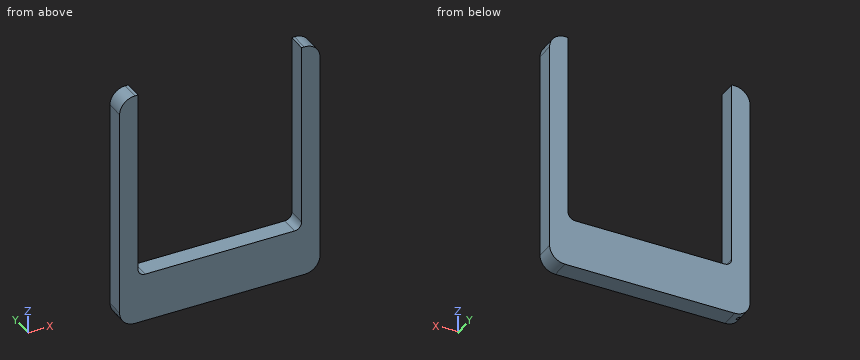
Autodesk Fusion 360 part; units mm, degrees
sketch "Sketch1" plane through (0, 0, 0) normal (0, 1, 0) x (1, 0, 0)
  line L0 (-207.5, 295) -> (207.5, 295)
  line L1 (245, 257.5) -> (245, -257.5)
  line L2 (-245, -257.5) -> (-245, 257.5)
  arc A0 (-207.5, 295) -> (-245, 257.5) centre (-207.5, 257.5) ccw
  arc A1 (245, 257.5) -> (207.5, 295) centre (207.5, 257.5) ccw
  arc A2 (207.5, -295) -> (245, -257.5) centre (207.5, -257.5) ccw
  arc A3 (-245, -257.5) -> (-207.5, -295) centre (-207.5, -257.5) ccw
  line L3 (-207.5, -295) -> (207.5, -295)
  line L4 (-207.5, 257.5) -> (207.5, -257.5) construction
  line L5 (-207.5, -257.5) -> (207.5, 257.5) construction
  point P0 (-245, 295)
  point P1 (245, 295)
  point P2 (-245, -523.5619)
  dimension "d2" = 490
  dimension "d6" = 37.5
  dimension "d10" = 590
extrude "Extrude1" add sketch "Sketch1" along normal blind 4
equation "d2 = 400 mm + 45 mm + 45 mm"
equation "d10 = 500.00 mm + 45 mm + 45 mm"

Autodesk Fusion 360 part; units mm, degrees
sketch "Sketch1" plane through (0, 0, 0) normal (0, 1, 0) x (1, 0, 0)
  line L0 (0, 0) -> (35, 0)
  line L1 (35, 0) -> (0, -35)
  line L2 (0, -35) -> (0, 0)
  dimension "d1" = 35
  dimension "d2" = 35
extrude "Extrude1" add sketch "Sketch1" along normal blind 45
sketch "Sketch2" plane through (0, 0, 0) normal (-1, 0, 0) x (0, 0, 1)
  line L0 (0, 0) -> (35, 0)
  line L1 (35, 0) -> (35, 45)
  line L2 (35, 45) -> (0, 45)
  line L3 (0, 45) -> (0, 0)
  line L4 (0, 45) -> (35, 0) construction
  circle A0 centre (17.5, 22.5) radius 4.5
  dimension "d5" = 9
extrude "Extrude2" cut sketch "Sketch2" against normal blind 110 contours A0
sketch "Sketch3" plane through (0, 0, 0) normal (0, 0, -1) x (-1, 0, 0)
  line L0 (-35, 0) -> (0, 0)
  line L1 (0, 0) -> (0, 45)
  line L2 (0, 45) -> (-35, 45)
  line L3 (-35, 45) -> (-35, 0)
  line L4 (0, 45) -> (-35, 0) construction
  circle A0 centre (-17.5, 22.5) radius 4.5
  point P0 (0, 22.5)
  dimension "d8" = 9
extrude "Extrude3" cut sketch "Sketch3" against normal blind 45 contours A0
sketch "Sketch4" plane through (0, 0, 0) normal (0, 0, -1) x (-1, 0, 0)
  circle A0 centre (-17.5, 22.5) radius 4.5
  line L0 (-35, 0) -> (0, 0)
  line L1 (0, 0) -> (0, 45)
  line L2 (0, 45) -> (-35, 45)
  line L3 (-35, 45) -> (-35, 0)
  point P0 (0, 22.5)

Autodesk Fusion 360 part; units mm, degrees
sketch "Sketch1" plane through (0, 0, 0) normal (0, 1, 0) x (1, 0, 0)
  line L0 (37.5, 0) -> (452.5, 0)
  line L1 (490, -37.5) -> (490, -552.7439)
  line L2 (0, -552.5) -> (0, -37.5)
  line L3 (445, -590) -> (445, -137.5)
  line L4 (427.5, -120) -> (62.5, -120)
  line L5 (45, -137.5) -> (45, -590)
  arc A0 (37.5, 0) -> (0, -37.5) centre (37.5, -37.5) ccw
  arc A1 (490, -37.5) -> (452.5, 0) centre (452.5, -37.5) ccw
  arc A2 (451.1619, -590.22) -> (490, -552.7439) centre (452.5, -552.7439) ccw
  arc A3 (0, -552.5) -> (37.5, -590) centre (37.5, -552.5) ccw
  arc A4 (62.5, -120) -> (45, -137.5) centre (62.5, -137.5) ccw
  arc A5 (445, -137.5) -> (427.5, -120) centre (427.5, -137.5) ccw
  line L6 (445, -590) -> (451.1619, -590.22)
  line L7 (37.5, -590) -> (45, -590)
  point P0 (490, 0)
  dimension "d1" = 45
  dimension "width" = 490
  dimension "d4" = 45
  dimension "d5" = 120
  dimension "d6" = 37.5
  dimension "d9" = 17.5
  dimension "length" = 590
  dimension "d11" = 590
extrude "Extrude1" add sketch "Sketch1" along normal blind 4
ref_plane "WorkPlane1" through (245, 0, 0) normal (1, 0, 0) x (0, 1, 0)
equation "width = 400 mm + 45 mm + 45 mm"
equation "length = 500.00 mm + 45 mm + 45 mm"
equation "d11 = length"
equation "d12 = width / 2"
Verification items for the finished model (mm, model axes). Coordinates: 2 decimals unless noted, no trailing zeros. Loops run counter-clockwise (first coordinate to the right, second up) from the corner with the lowest first, then second, coordinate; pieces in that order, holes last. Notation, with made-up numbers: (15.25, 73) -> (26.25, 73) arc R15 ccw to (26.25, 85) -> close; hole circle Ø5 at (64, 42). An arc over 180 degrees is marked (long way). Answer as CSV lines item,"result".
1) Cross-section at B-B, the plane x = 359. Record the cut outline in (y, z), then the cut area to 3 significant figures.
Found:
outline,"(0, 0) -> (45, 0) -> (45, 120) -> (0, 120) -> close"
area,"5,400 mm2"
2) Cross-section at A-A, the plane z = 364. Record the cut outline in (x, y), then the cut area to 3 significant figures.
Found:
outline,"(0, 0) -> (45, 0) -> (45, 45) -> (0, 45) -> close; (445, 0) -> (490, 0) -> (490, 45) -> (445, 45) -> close"
area,"4,050 mm2"
3) Thickness scan on L1, parallel to X at y = 4.5, z = 442; L2, parallel to X at y = 22.5, z = 34.25; L3, parallel to Y at x = 14, z = 17. Record the ranges inside material, lowest first. Write a range as from..to.
Found:
L1,"x = 0..45, 445..490"
L2,"x = 0.14..13, 22..489.86"
L3,"y = 0..18.03, 26.97..45"
4) Depth check by flat-ended pin: pin 1 (10 mm diameter, centred on y = 21.5, z = 16.5, fed in from -X); pin 2 (10.5 mm diameter, centred on y = 22.5, z = 17.5, fed in from -X); pin 3 (10 mm diameter, centred on x = 170, y = 34.5, fed in from +Z). Enter the tip coordinate at first touch or a pass-through.
Found:
pin 1,"stops at x = 3.68"
pin 2,"stops at x = 3.02"
pin 3,"stops at z = 120"
